Autodesk Inventor part; units mm, degrees
ref_plane "YZ Plane" through (0, 0, 0) normal (1, 0, 0) x (0, 1, 0)
ref_plane "XZ Plane" through (0, 0, 0) normal (0, 1, 0) x (-1, 0, 0)
ref_plane "XY Plane" through (0, 0, 0) normal (0, 0, 1) x (1, 0, 0)
sketch "Sketch1" plane through (0, 0, 0) normal (0, 0, 1) x (1, 0, 0)
  circle A0 centre (0, 0) radius 3.175
  dimension "d0" = 6.35
extrude "Extrusion1" add sketch "Sketch1" along normal blind 89.408
hole "Hole2" at (0, 0, 0) direction (0, 0, 1) diameter 4.0132 depth 29.21 tip angle 118 countersink diameter 4.5212 countersink angle 90
chamfer "Chamfer3" distance 0.381 angle 45 2 edges at (-3.175, 0, 89.408) (-3.175, 0, 0)
sketch "Sketch11" plane through (0, 0, 0) normal (1, 0, 0) x (0, 1, 0)
  line L0 (-2.0066, 29.21) -> (2.0066, 29.21)
  line L1 (0, 107.2896) -> (0, -17.8816)
  circle A0 centre (0, 28.448) radius 0.762 construction
  point P0 (0, 0)
  dimension "d65" = 1.524
hole "Hole3" at (0, 0, 28.448) direction (-1, 0, 0) diameter 1.524 depth 3.81 tip angle 118
properties part number "J008574 NEUROPIXELS GEN 2 ROD ADAPTER Rev -" material "ALUMINUM, 6061-T651"
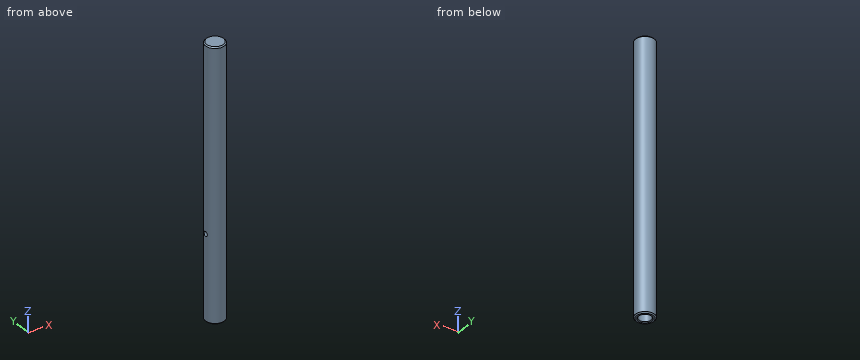
The model under review builds one solid part; all positions refer to its coordinate system, in mm. Round coordinates to 2 decimals unless told otherwise and drop trailing zeros. Loops run counter-clockwise (first coordinate to the right, second up) from the corner with the lowest first, then second, coordinate; pieces in that order, holes last. Notation, with made-up numbers: M 7.25,34 L 34.25,34 A11 ccw 34.25,47 Z; hole C -13.75,-16.75 d7. An arc over 180 degrees is marked long. Answer as a JSON object with one key per item and string values.
Item 1: We need section A-A, the plane z = 65. State the section outline as (x, y) points (3 decimals), and give its area (3 significant figures).
Check sheet entries:
{"outline": "C 0,0 d6.35", "area": "31.7 mm2"}
Item 2: Clearance check with flat-ended pins moving along their axes: P1, Ø1, axis at y = 1, z = 16, coming from the +X side; P2, Ø1.5, axis at x = -1, z = 43, coming from the +Y side; P3, Ø1.5, axis at x = -1.5, z = 9.5, coming from the +Y side. State where each tip first meets the part, or that it passes through.
Check sheet entries:
{"P1": "x = 3.14", "P2": "y = 3.17", "P3": "y = 3.09"}
Item 3: For line 1 along Y through (x, z) = (0, 7) (3 decimals); line 2 along Z through (x, y) = (-2.6, 0), list the stretches that pass through material, from the lowest coordinate up.
Check sheet entries:
{"line 1": "-3.175 to -2.007, 2.007 to 3.175", "line 2": "0 to 27.69, 29.21 to 89.41"}
